from build123d import *

# Parameters (mm, degrees)
F0_R      = 11.938
F1_DEPTH  = 14.986
F2_R      = 5.2835878492
F3_DEPTH  = 6.35
F4_W      = 26.416
F4_H      = 30.734
F5_DEPTH  = 28.956
F6_R      = 0.635
F7_DEPTH  = 6.35
F8_R      = 0.635
F9_DEPTH  = 6.35
F10_R     = 6.35
F11_DEPTH = 14.986
F13_R     = 2.032
F14_W     = 0.381
F14_H     = 1.27
F15_DEPTH = 0.254


with BuildPart() as f1:
    # F0 (on Top) → F1 (new body)
    with BuildSketch(Plane.XY):
        Circle(F0_R)
    extrude(amount=F1_DEPTH)

    # F2 (on face) → F3 (cut)
    with BuildSketch(Plane.XY.offset(14.986)):
        Circle(F2_R)
    extrude(amount=-F3_DEPTH, mode=Mode.SUBTRACT)


with BuildPart() as f5:
    # F4 (on Top) → F5 (new body)
    with BuildSketch(Plane.XY):
        with Locations((54.4431246817, 16.2993484654)):
            Rectangle(F4_W, F4_H)
    extrude(amount=F5_DEPTH)

    # F6 (on face) → F7 (cut)
    with BuildSketch(Plane(origin=(41.2351246817, 0, 0), x_dir=(0, -1, 0), z_dir=(-1, 0, 0))):
        with Locations((-7.2823484654, 25.654)):
            Circle(F6_R)
    extrude(amount=-F7_DEPTH, mode=Mode.SUBTRACT)

    # F8 (on face) → F9 (cut)
    with BuildSketch(Plane.YZ.offset(67.6511246817)):
        with Locations((28.1103484654, 25.654)):
            Circle(F8_R)
    extrude(amount=-F9_DEPTH, mode=Mode.SUBTRACT)

    # F10 (on face) → F11 (join)
    with BuildSketch(Plane.XY.offset(28.956)):
        with BuildLine():
            ThreePointArc((57.908611975, 0.9323484654), (64.7262122314, 5.0905971842), (67.3971246817, 12.6163484654))
            ThreePointArc((67.3971246817, 12.6163484654), (47.9333734005, 21.8834360151), (53.0096373884, 0.9323484654))
            Line((53.0096373884, 0.9323484654), (57.908611975, 0.9323484654))
        make_face()
        with Locations((55.4591246817, 12.6163484654)):
            Circle(F10_R, mode=Mode.SUBTRACT)
        with BuildLine():
            Line((57.908611975, 0.9323484654), (53.0096373884, 0.9323484654))
            ThreePointArc((53.0096373884, 0.9323484654), (55.4591246817, 0.6783484654), (57.908611975, 0.9323484654))
        make_face()
    extrude(amount=F11_DEPTH)

    # F13
    f13_edges = [f5.edges().sort_by_distance(p)[0] for p in [
        (41.235125, 31.666348, 14.478),
        (67.651125, 31.666348, 14.478),
        (41.235125, 0.932348, 14.478),
        (67.651125, 0.932348, 14.478),
    ]]
    fillet(f13_edges, radius=F13_R)

    # F14 (on face) → F15 (cut)
    with BuildSketch(Plane(origin=(41.2351246817, 0, 0), x_dir=(0, -1, 0), z_dir=(-1, 0, 0))):
        Polygon((-17.3889424292, 3.302), (-17.3889424292, 2.032), (-9.7689424292, 2.032), (-9.7689424292, 3.302), (-9.7689424292, 4.572), (-9.7689424292, 7.112), (-17.3889424292, 7.112), (-17.3889424292, 4.572), align=None)
        with Locations((-17.5794424292, 2.667)):
            Rectangle(F14_W, F14_H)
        Polygon((-17.7699424292, 3.302), (-17.3889424292, 3.302), (-17.3889424292, 4.572), align=None)
        Polygon((-9.7689424292, 4.572), (-9.7689424292, 3.302), (-9.3879424292, 3.302), align=None)
        with Locations((-9.5784424292, 2.667)):
            Rectangle(F14_W, F14_H)
    extrude(amount=-F15_DEPTH, mode=Mode.SUBTRACT)


solid = f5.part
Work out the finished part from the listing and answer in its coordinate system (mm). A direction names the side the tool comes from. Coordinates: 2 decimals unless noted, no trailing zeros. Write each loop counter-clockwise with the first axis right and the second up, starting at its lowest first coordinate (ties: lowest second). Pieces come first, ordered by that corner, then holes.
1. The part is cut by section D-D, the plane x = 56.75. Write down the section's boundary in (y, z), and give its area (3 significant figures).
Results list:
outline: (0.75, 28.96) - (0.93, 28.96) - (0.93, 0) - (31.67, 0) - (31.67, 28.96) - (24.48, 28.96) - (24.48, 43.94) - (18.83, 43.94) - (18.83, 28.96) - (6.4, 28.96) - (6.4, 43.94) - (0.75, 43.94) - close
area: 1,060 mm2
2. The part is cut by section A-A, the plane x = 62.5. Write down the section's boundary in (y, z) (3 decimals), and give its area (3 significant figures).
Results list:
outline: (0.932, 0) - (31.666, 0) - (31.666, 28.956) - (22.257, 28.956) - (22.257, 43.942) - (2.976, 43.942) - (2.976, 28.956) - (0.932, 28.956) - close; hole circle Ø1.27 at (28.11, 25.654)
area: 1,180 mm2
3. Flat-ended cylindrical pins translate along their axes: pin 1 (4 mm diameter, centred on x = 53.5, y = 13, fed in from +Z); pin 2 (6.5 mm diameter, centred on x = 49.5, z = 14.5, fed in from -Y); pin 3 (5 mm diameter, centred on x = 57, z = 37.5, fed in from +Y). Find the tip coordinate at first contact, or state that the pin passes through.
Results list:
pin 1: stops at z = 28.96
pin 2: stops at y = 0.93
pin 3: stops at y = 24.55
4. Consider line 1 along X through (y, z) = (12.5, 37); line 2 along Y through (x, z) = (45.25, 28); line 3 along Z through (x, y) = (50.75, 27). Determine where each line is inside the solid, lowest interval first.
Results list:
line 1: x = 43.52 to 49.11, 61.81 to 67.4
line 2: y = 0.93 to 31.67
line 3: z = 0 to 28.96
5. For a pull along Z with two mould halves and no side action, classify faces 1 (the flat face through (55, 13, 28.956)), 2 (the cylindrical face through (64.521, 27.476, 25.682)), 3 (the flat face through (61.301, 28, 26)), 4 (the cylindrical face through (67.07, 1.54, 14.68)) as +Z half, -Z half, draft (parallel to the pull), parting line (faces both ways), or undercut.
Results list:
face 1: +Z half
face 2: undercut
face 3: undercut
face 4: draft
6. The part is cut by section C-C, the plane z = 34. Write down the section's boundary in (x, y).
Results list:
outline: circle Ø23.88 at (55.46, 12.62); hole circle Ø12.7 at (55.46, 12.62)
7. The part is cut by section B-B, the plane y = 20. Write down the section's boundary in (x, z).
Results list:
outline: (41.24, 0) - (67.65, 0) - (67.65, 28.96) - (64.84, 28.96) - (64.84, 43.94) - (46.08, 43.94) - (46.08, 28.96) - (41.24, 28.96) - close
8. For faces 5 (the flat face through (47.585, 7, 26)), 6 (the flat face through (48, 23, 28.956)), 7 (the flat face through (54, 0.932, 14)), determine the directions among +Z, -Z, +X, -X, +Y, -Y from which every point of the face is accessible in a straight line to the end or side of a thin tool.
Results list:
face 5: -X
face 6: +Z
face 7: -Z, +X, -X, -Y
